Can you work these out from the model? Positions are in its coordinate system, mm. A direction names the side the tool comes from. Coordinates: 2 decimals unless noted, no trailing zeros. Write each loop counter-clockwise with the first axis right and the second up, starting at its lowest first coordinate (ties: lowest second). Pieces come first, ordered by that corner, then holes. Notation, with made-up numbers: M -20,24 L 39,24 A15 cw 39,45 Z; hole C 44.25,4.5 d9. An arc over 180 degrees is marked long. Answer as a JSON object with one key per item and string values. Group by question number.
from build123d import *

# Parameters (mm, degrees)
F0_R     = 2
F1_DEPTH = 19
F2_R     = 3
F3_R     = 10
F4_R     = 2.5
F5_R     = 1
F6_R     = 1


with BuildPart() as f1:
    # F0 (on Top) → F1 (new body)
    with BuildSketch(Plane.XY):
        with BuildLine():
            Line((0, 24), (0, 0))
            Line((0, 0), (4, 0))
            ThreePointArc((4, 0), (5.209430585, 3.8717082451), (8.5, 1.5))
            ThreePointArc((8.5, 1.5), (8.3717082451, 0.709430585), (8, 0))
            Line((8, 0), (12, 0))
            Line((12, 0), (12, 14))
            Line((12, 14), (12, 24))
            Line((12, 24), (9.8445055786, 24))
            Line((9.8445055786, 24), (0, 24))
        make_face()
        with Locations((6, 19)):
            Circle(F0_R, mode=Mode.SUBTRACT)
        with BuildLine():
            ThreePointArc((44.5191347039, 18.2475463293), (29.1095626147, 32.7438155226), (9.8445055786, 24))
            Line((9.8445055786, 24), (12, 24))
            Line((12, 24), (12, 14))
            ThreePointArc((12, 14), (24.9974259249, 27.964055472), (39.8564064606, 16))
            Line((39.8564064606, 16), (44.5191347039, 18.2475463293))
        make_face()
    extrude(amount=F1_DEPTH)

    # F2
    f2_edges = [f1.edges().sort_by_distance(p)[0] for p in [
        (0, 24, 9.5),
    ]]
    fillet(f2_edges, radius=F2_R)

    # F3
    f3_edges = [f1.edges().sort_by_distance(p)[0] for p in [
        (9.844506, 24, 9.5),
    ]]
    fillet(f3_edges, radius=F3_R)

    # F4
    f4_edges = [f1.edges().sort_by_distance(p)[0] for p in [
        (44.519135, 18.247546, 9.5),
    ]]
    fillet(f4_edges, radius=F4_R)

    # F5
    f5_edges = [f1.edges().sort_by_distance(p)[0] for p in [
        (39.856406, 16, 9.5),
    ]]
    fillet(f5_edges, radius=F5_R)

    # F6
    f6_edges = [f1.edges().sort_by_distance(p)[0] for p in [
        (4, 0, 9.5),
        (8, 0, 9.5),
    ]]
    fillet(f6_edges, radius=F6_R)


solid = f1.part
Q1. On a 3-axis mill with a long thin cutter (end or side, diameter ignored), from which of +Z, -Z, +X, -X, +Y, -Y can I reach the whole of each face in a straight line? I mean faces 1 (the flat face through (12, 7, 9)), 2 (the cylindrical face through (43.85, 18.66, 9.63)). Say none if no direction works.
Q2. If we section it at B-B on x = 6: List the corners of the cut face in (y, z) for me.
Q3. Please list where these lines run through material, in increasing order: L1, parallel to X at y = 20, z = 6.25; L2, parallel to X at y = 3, z = 17.75; L3, parallel to X at y = 6.5, z = 14.
Q4. If we section it at A-A on y = 24.5: List the corners of the cut face in (x, z) for me.
Q5. Will these pins go through, and if not, where does the flat tip stop? pin 1 (1 mm diameter, centred on x = 4, z = 13.5, fed in from +Y); pin 2 (6 mm diameter, centred on x = 39.5, z = 10.5, fed in from +Y); pin 3 (2.5 mm diameter, centred on x = 6, y = 19, fed in from -Z); pin 4 (2 mm diameter, centred on x = 7.5, z = 10, fed in from +Y).
Q6. If we section it at C-C on y = 19.5: List the corners of the cut face in (x, z) for me, and give its area (3 significant figures).
Q7. If we section it at D-D on z = 2.5: List the corners of the cut face in (x, y) for me.
Q8. We'd pull the mould along X, two halves only. Please class faces 3 (the flat face through (4, 24, 9)), 4 (the cylindrical face through (8.716, 0.336, 9.633)), 5 (the cylindrical face through (0.86, 23.1, 9.63)), 6 (the cylindrical face through (30.188, 32.533, 9.367)): pulls with the +X half, pulls with the -X half, needs draft (parallel to the pull), parting line crosses it, or undercut.
Reply:
{
 "1": {"face 1": "+Z, -Z, +X, -Y", "face 2": "+Z, -Z, +X"},
 "2": {"outline": "M 4,0 L 17,0 L 17,19 L 4,19 Z; M 21,0 L 24.05,0 L 24.05,19 L 21,19 Z"},
 "3": {"L1": "0 to 4.27, 7.73 to 13.35, 38.65 to 43.99", "L2": "0 to 4, 8 to 12", "L3": "0 to 12"},
 "4": {"outline": "M 8.12,0 L 16.74,0 L 16.74,19 L 8.12,19 Z; M 35.26,0 L 41.84,0 L 41.84,19 L 35.26,19 Z"},
 "5": {"pin 1": "y = 24", "pin 2": "y = 29.84", "pin 3": "through", "pin 4": "y = 24.63"},
 "6": {"outline": "M 0,0 L 4.06,0 L 4.06,19 L 0,19 Z; M 7.94,0 L 13.13,0 L 13.13,19 L 7.94,19 Z; M 38.87,0 L 44.03,0 L 44.03,19 L 38.87,19 Z", "area": "274 mm^2"},
 "7": {"outline": "M 0,0 L 2.54,0 A1 ccw 3.53,1.14 A2.5 cw long 8.47,1.14 A1 ccw 9.46,0 L 12,0 L 12,14 A14 cw 39.62,17.23 A1 ccw 41.03,16.56 L 42.61,17.33 A2.5 ccw 43.88,20.43 A19 ccw 12.24,27.1 A10 cw 5,24 L 3,24 A3 ccw 0,21 Z; hole C 6,19 d4"},
 "8": {"face 3": "needs draft", "face 4": "undercut", "face 5": "pulls with the -X half", "face 6": "parting line crosses it"}
}
